Source: CAD feature listing. Evaluate the final solid. Frame: model axes, mm. A direction names the side the tool comes from. Coordinates: 2 decimals unless noted, no trailing zeros. Order: outer loops, then holes, each group sorted by start corner. A loop starts at its lowest first (then second) coordinate and runs counter-clockwise, first axis right, second up.
```python
from build123d import *

# Parameters (mm, degrees)
BOSS_EXTRUDE1_DEPTH = 22.4
SKETCH2_R           = 14
BOSS_EXTRUDE2_DEPTH = 150
CHAMFER1_SIZE       = 2.8
SKETCH3_OUTSIDE_W   = 607.642
SKETCH3_OUTSIDE_H   = 615.144
SKETCH3_OUTSIDE_R   = 24.248711306
CUT_EXTRUDE1_DEPTH  = 150
CUT_EXTRUDE1_TAPER  = 60


with BuildPart() as part:
    # Sketch1 → Boss-Extrude1 (new body)
    with BuildSketch(Plane(origin=(0, 0, 0), x_dir=(0, 0, -1), z_dir=(1, 0, 0))):
        Polygon((0, 28), (-24.248711306, 14), (-24.248711306, -14), (0, -28), (24.248711306, -14), (24.248711306, 14), align=None)
    extrude(amount=-BOSS_EXTRUDE1_DEPTH)

    # Sketch2 → Boss-Extrude2 (add)
    with BuildSketch(Plane(origin=(0, 0, 0), x_dir=(0, 0, -1), z_dir=(1, 0, 0))):
        Circle(SKETCH2_R)
    extrude(amount=BOSS_EXTRUDE2_DEPTH)

    # Chamfer1
    chamfer1_edges = [part.edges().sort_by_distance(p)[0] for p in [
        (150, 0, 14),
    ]]
    chamfer(chamfer1_edges, length=CHAMFER1_SIZE)

    # Sketch3 outside → Cut-Extrude1 (cut)
    with BuildSketch(Plane.ZY.offset(22.4)):
        Rectangle(SKETCH3_OUTSIDE_W, SKETCH3_OUTSIDE_H)
        Circle(SKETCH3_OUTSIDE_R, mode=Mode.SUBTRACT)
    extrude(amount=-CUT_EXTRUDE1_DEPTH, taper=CUT_EXTRUDE1_TAPER, mode=Mode.SUBTRACT)


solid = part.part
```
1. Pin query (flat end, axial travel): P1, Ø6, axis at x = 17, z = 2, coming from the -Y side; P2, Ø2, axis at x = 104, z = -13, coming from the +Y side; P3, Ø5, axis at x = 36.5, z = -5.5, coming from the -Y side. Return the tip coordinate at first contact, or that it passes through.
Findings:
P1: stops at y = -14
P2: stops at y = 7.21
P3: stops at y = -13.67
2. Section query A-A on x = -4. Return loops of the section in (y, z), plus the area to 3 significant figures.
Findings:
outline: (-28, 0) - (-14, -24.25) - (14, -24.25) - (28, 0) - (14, 24.25) - (-14, 24.25) - close
area: 2,040 mm2
3. Ray query, line 1 (X direction, y = 16.5, z = -1); line 2 (Z direction, x = 140, y = -7.5); line 3 (Z direction, x = 40, y = 13). Return the intervals inside material, ascending.
Findings:
line 1: x = -22.4 to 0
line 2: z = -11.82 to 11.82
line 3: z = -5.2 to 5.2
4. Access query for faces 1 (the face through (72.57, -5.362, -12.932)), 2 (the face through (-21.874, -12.527, 21.82)). Directions: +Z, -Z, +X, -X, +Y, -Y. A direction counts if a zero-diameter tool reaches every point of the face in a straight line with its end or side. Return the directions, or none.
Findings:
face 1: +X
face 2: +Z, -X, -Y
5. Section query B-B on x = 103.5. Return loops of the section in (y, z).
Findings:
outline: circle Ø28 at (0, 0)
